Part model, mm, in its own coordinate system. Face numbers are marked on the shaded views. A direction names the side the tool comes from. Coordinates: 2 decimals unless noted, no trailing zeros. Loops run counter-clockwise (first coordinate to the right, second up) from the corner with the lowest first, then second, coordinate; pieces in that order, holes last. Notation, with made-up numbers: (78, -9) - (107, -9) arc R23 cw to (107, 23) - close; hole circle Ø3 at (71.25, -35.75). An arc over 180 degrees is marked (long way). Answer as CSV lines item,"result".
Autodesk Inventor part; units mm, degrees
ref_plane "YZ Plane" through (0, 0, 0) normal (1, 0, 0) x (0, 1, 0)
ref_plane "XZ Plane" through (0, 0, 0) normal (0, 1, 0) x (-1, 0, 0)
ref_plane "XY Plane" through (0, 0, 0) normal (0, 0, 1) x (1, 0, 0)
sketch "Sketch1" plane through (0, 0, 0) normal (1, 0, 0) x (0, 1, 0)
  line L0 (0, 0) -> (114.3, 0)
  line L1 (114.3, 0) -> (114.3, -139.7)
  line L2 (114.3, -139.7) -> (0, -139.7)
  line L3 (0, -139.7) -> (0, 0)
  line L4 (111.125, -136.525) -> (111.125, -3.175)
  line L5 (111.125, -3.175) -> (3.175, -3.175)
  line L6 (3.175, -3.175) -> (3.175, -136.525)
  line L7 (3.175, -136.525) -> (111.125, -136.525)
  dimension "d0" = 114.3
  dimension "d1" = 139.7
  dimension "d2" = 3.175
extrude "Extrusion1" add sketch "Sketch1" along normal blind 215.9
sketch "Sketch2" plane through (0, 0, 0) normal (0, 0, 1) x (1, 0, 0)
  line L0 (215.9, 114.3) -> (177.8, 114.3)
  line L1 (177.8, 114.3) -> (177.8, 3.175)
  line L2 (177.8, 3.175) -> (215.9, 3.175)
  line L3 (215.9, 3.175) -> (215.9, 114.3)
  point P0 (0, 0)
  dimension "d5" = 38.1
  dimension "d6" = 111.125
extrude "Extrusion2" cut sketch "Sketch2" against normal through all
sketch "Sketch4" plane through (0, 0, 0) normal (0, 0, 1) x (1, 0, 0)
  line L0 (177.8, 3.175) -> (177.8, 114.3)
  line L1 (0, 114.3) -> (177.8, 114.3)
  circle A0 centre (127, 97.79) radius 4
  line L2 (127, 97.79) -> (134.9404, 98.765)
  line L3 (127, 97.79) -> (135, 97.79) construction
  line L4 (127, 97.79) -> (126.025, 105.7304)
  circle A1 centre (126.025, 105.7304) radius 1.85
  circle A2 centre (134.9404, 98.765) radius 1.85
  dimension "d13" = 50.8
  dimension "d14" = 16.51
  dimension "d15" = 8
  dimension "d16" = 8
  dimension "d17" = 353
  dimension "d18" = 8
  dimension "d19" = 3.7
  dimension "d20" = 3.7
  dimension "d23" = 90
extrude "Extrusion3" cut sketch "Sketch4" against normal blind 25.4 contours A1 | A2
properties part number "Bucket" material "Polycarbonate, Clear"
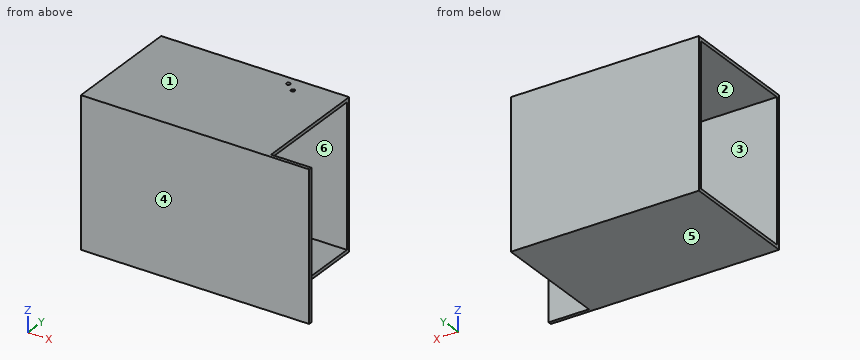
Q1. Saw through at C-C (x = 52.5). Give the cut face in (y, z) (3 decimals), then the cut area to 3 significant figures.
Results:
outline,"(0, -139.7) - (114.3, -139.7) - (114.3, 0) - (0, 0) - close; hole (3.175, -136.525) - (111.125, -136.525) - (111.125, -3.175) - (3.175, -3.175) - close"
area,"1,570 mm^2"
Q2. Two-plate mould, pull along Z, no slides. Class the marked faces 1, 2, 3 and 4: released by +Z, released by -Z, zero draft, split by the parting line, or undercut.
Results:
face 1,"released by +Z"
face 2,"undercut"
face 3,"undercut"
face 4,"zero draft"
Q3. Saw through at B-B (z = -119.5). Give the cut face in (x, y) (3 decimals), then the cut area to 3 significant figures.
Results:
outline,"(0, 0) - (215.9, 0) - (215.9, 3.175) - (0, 3.175) - close; (0, 111.125) - (177.8, 111.125) - (177.8, 114.3) - (0, 114.3) - close"
area,"1,250 mm^2"
Q4. Which spindle directions (+Z, -Z, +X, -X, +Y, -Y) get a long thin tool onto all of the face, cutting with end or side? Do the marked faces 5 and 6. Say none if no direction does.
Results:
face 5,"-Z, +X, -X, +Y, -Y"
face 6,"+X, -X"
Q5. Saw through at D-D (x = 197.5). Give the cut face in (y, z) (3 decimals), then the cut area to 3 significant figures.
Results:
outline,"(0, -139.7) - (3.175, -139.7) - (3.175, 0) - (0, 0) - close"
area,"444 mm^2"
Q6. Wall check: L1, parallel to Y at x = 142, z = -70 (3 decimals); L2, parallel to Z at x = 172.5, y = 17 (3 decimals); L3, parallel to Y at x = 200.5, z = -109.5 (3 decimals). Give the ranges that are in metal, low to high.
Results:
L1,"y = 0 to 3.175, 111.125 to 114.3"
L2,"z = -139.7 to -136.525, -3.175 to 0"
L3,"y = 0 to 3.175"
Q7. Saw through at A-A (y = 38). Give the cut face in (x, z) (3 decimals).
Results:
outline,"(0, -139.7) - (177.8, -139.7) - (177.8, -136.525) - (0, -136.525) - close; (0, -3.175) - (177.8, -3.175) - (177.8, 0) - (0, 0) - close"
